Build history of the part. All positions in model axes, mm. A direction names the side the tool comes from. Coordinates: 2 decimals unless noted, no trailing zeros. Write each loop counter-clockwise with the first axis right and the second up, starting at its lowest first coordinate (ties: lowest second). Pieces come first, ordered by that corner, then holes.
```python
from build123d import *

# Parameters (mm, degrees)
SKETCH1_R               = 60
BOSS_EXTRUDE1_DEPTH     = 10
SKETCH2_R               = 10
BOSS_EXTRUDE2_DEPTH     = 30
SKETCH3_R               = 3.18
CUT_EXTRUDE1_DEPTH      = 30
CUT_EXTRUDE2_REACH      = 106.043
CUT_EXTRUDE2_END_RADIUS = 3.18
SKETCH4_R               = 1.5


with BuildPart() as part:
    # Sketch1 → Boss-Extrude1 (new body)
    with BuildSketch(Plane.XY):
        Circle(SKETCH1_R)
    extrude(amount=BOSS_EXTRUDE1_DEPTH)

    # Sketch2 → Boss-Extrude2 (add)
    with BuildSketch(Plane.XY.offset(10)):
        Circle(SKETCH2_R)
    extrude(amount=BOSS_EXTRUDE2_DEPTH)

    # Sketch3 → Cut-Extrude1 (cut)
    with BuildSketch(Plane.XY.offset(40)):
        Circle(SKETCH3_R)
    extrude(amount=-CUT_EXTRUDE1_DEPTH, mode=Mode.SUBTRACT)

    # Cut-Extrude2: up to this cylinder (the profile starts outside it)
    cut_extrude2_end = Plane(origin=(0, 0, 32), z_dir=(0, 0, 1)) * Cylinder(CUT_EXTRUDE2_END_RADIUS, 219.446, mode=Mode.PRIVATE)
    # Sketch4 → Cut-Extrude2 (cut, up to the surface)
    with BuildSketch(Plane(origin=(0, 15, 0), x_dir=(1, 0, 0), z_dir=(0, 1, 0)), mode=Mode.PRIVATE) as cut_extrude2_sk1:
        with Locations(Location((0, -32, 0), (0, 0, 270))):
            Circle(SKETCH4_R)
    cut_extrude2_tool1 = extrude(cut_extrude2_sk1.sketch, amount=-CUT_EXTRUDE2_REACH, mode=Mode.PRIVATE) - cut_extrude2_end
    add(cut_extrude2_tool1.solids().sort_by_distance((0, 15, 32))[0], mode=Mode.SUBTRACT)


solid = part.part
```
1. Flat gauge pins, fed straight in: pin 1 (2 mm diameter, centred on y = -9, z = 21, fed in from +X); pin 2 (12 mm diameter, centred on x = 36.5, z = 9, fed in from -Y); pin 3 (2.5 mm diameter, centred on x = 0, z = 32, fed in from -Y). Where does each tip first touch, or does it go through?
Computed values:
pin 1: stops at x = 6
pin 2: stops at y = -51.67
pin 3: stops at y = -10
2. Saw through at B-B on z = 12. List the corners of the cut face in (x, y), plus the area to 3 significant figures.
Computed values:
outline: circle Ø20 at (0, 0); hole circle Ø6.36 at (0, 0)
area: 282 mm2
3. Mould opens along X. For faces 1 (the face through (-0.7, -3.1, 25.2)), 2 (the face through (-2.17, -9.76, 24.79)), 3 (the face through (12, 1, 10)) say: +X half, -X half, draft (parallel to the pull), parting line (faces both ways), or undercut.
Computed values:
face 1: undercut
face 2: parting line
face 3: draft
4. Saw through at D-D on y = -24.5. List the corners of the cut face in (x, z).
Computed values:
outline: (-54.77, 0) - (54.77, 0) - (54.77, 10) - (-54.77, 10) - close
5. Probe line 1 along Y through (x, z) = (0, 28.5); line 2 along Z through (x, y) = (0, 6); line 3 along Z through (x, y) = (37, -12). List the from-to ranges inside material, lowest first.
Computed values:
line 1: y = -10 to -3.18, 3.18 to 10
line 2: z = 0 to 30.5, 33.5 to 40
line 3: z = 0 to 10
6. 3-axis set-ups, long thin cutter, end or side, ignore diameter. For faces 4 (the face through (0.07, 6.45, 30.5)), 5 (the face through (0, 0, 10)), 6 (the face through (-1, 1, 0)): which of +Z, -Z, +X, -X, +Y, -Y reach the whole face in a straight line?
Computed values:
face 4: +Y
face 5: +Z
face 6: -Z, +X, -X, +Y, -Y
7. Saw through at C-C on x = -23. List the corners of the cut face in (y, z), plus the area to 3 significant figures.
Computed values:
outline: (-55.42, 0) - (55.42, 0) - (55.42, 10) - (-55.42, 10) - close
area: 1,110 mm2
8. Saw through at A-A on y = 8.5. List the corners of the cut face in (x, z), plus the area to 3 significant figures.
Computed values:
outline: (-59.39, 0) - (59.39, 0) - (59.39, 10) - (5.27, 10) - (5.27, 40) - (-5.27, 40) - (-5.27, 10) - (-59.39, 10) - close; hole circle Ø3 at (0, 32)
area: 1,500 mm2
